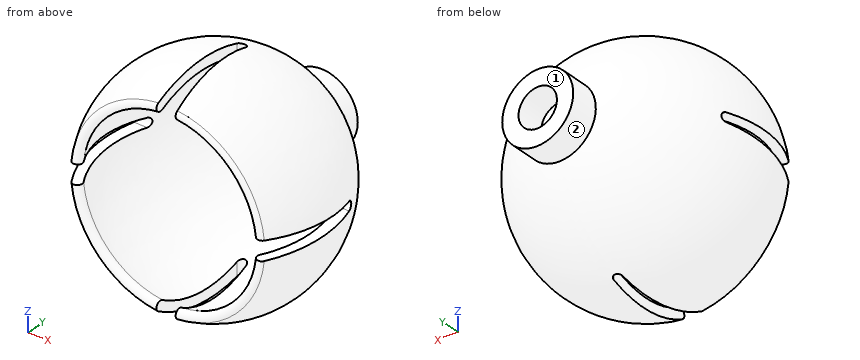
```python
from build123d import *

# Parameters (mm, degrees)
SKETCH1_R           = 3.7
SKETCH1_R_2         = 2
BOSS_EXTRUDE1_DEPTH = 3
CUT_EXTRUDE1_DEPTH  = 12.79718581
CIRPATTERN1_COUNT   = 4


with BuildPart() as part:
    # Sketch1 → Boss-Extrude1 (new body)
    with BuildSketch(Plane(origin=(0, 0, 0), x_dir=(1, 0, 0), z_dir=(0, 1, 0))):
        Circle(SKETCH1_R)
        Circle(SKETCH1_R_2, mode=Mode.SUBTRACT)
    extrude(amount=BOSS_EXTRUDE1_DEPTH)

    # Sketch2 → Revolve1 (revolve)
    with BuildSketch(Plane(origin=(0, 0, 0), x_dir=(0, 0, -1), z_dir=(1, 0, 0))):
        with BuildLine():
            Line((0, 0), (3.7, 0))
            ThreePointArc((3.7, 0), (11.06716667, -7.226007618), (10.1, -17.5))
            ThreePointArc((10.1, -17.5), (9.414366099, -17.672933956), (9.241432142, -16.987300055))
            ThreePointArc((9.241432142, -16.987300055), (9.596057225, -7.167858517), (1.5, -1.6))
            Line((1.5, -1.6), (1.5, -2.8))
            Line((1.5, -2.8), (0, -2.8))
            Line((0, -2.8), (0, 0))
        make_face()
    revolve(axis=Axis((0, 0, 0), (0, -1, 0)))

    # Sketch3 → Cut-Extrude1 (cut, symmetric)
    with BuildSketch(Plane(origin=(0, 0, 0), x_dir=(0, 0, -1), z_dir=(1, 0, 0))):
        with BuildLine():
            Line((-1, -17.743650027), (1, -17.743650027))
            Line((1, -17.743650027), (0.474618631, -7.718776319))
            ThreePointArc((0.474618631, -7.718776319), (0, -7.268380055), (-0.474618631, -7.718776319))
            Line((-0.474618631, -7.718776319), (-1, -17.743650027))
        make_face()
    cut_extrude1 = extrude(amount=CUT_EXTRUDE1_DEPTH, both=True, mode=Mode.SUBTRACT)

    # CirPattern1: Cut-Extrude1 ×4 about axis
    cirpattern1_axis = Axis((0, 0, 0), (0, 1, 0))
    for i in range(1, CIRPATTERN1_COUNT):
        add(cut_extrude1.rotate(cirpattern1_axis, i * 360 / CIRPATTERN1_COUNT), mode=Mode.SUBTRACT)


solid = part.part
```
Build history of the part. All positions in model axes, mm. Face numbers are marked on the shaded views. A direction names the side the tool comes from. Give positions to 0.01 mm unless a question says otherwise; leave off trailing zeros. Use a Markdown table: item, result.
(1) Wall check: line 1 along X through (y, z) = (2.3, 0); line 2 along Z through (x, y) = (-6.5, -7.75). Give the ranges that are in metal, low to high.
Taken from the geometry:
| item | result |
|---|---|
| line 1 | -3.7 to -2, 2 to 3.7 |
| line 2 | -9.18 to -7.42, 7.42 to 9.18 |
(2) Band-saw the part on A-A (y = -14.5). Give the number of separate pieces and of enclosed holes in the cut face, and give its area (3 significant figures).
Taken from the geometry:
| item | result |
|---|---|
| separate pieces | 4 |
| enclosed holes | 0 |
| area | 65.6 mm2 |
(3) Which spindle directions (+Z, -Z, +X, -X, +Y, -Y) get a long thin tool onto all of the face, cutting with end or side? Do the marked faces 1 and 2. Say none if no direction does.
Taken from the geometry:
| item | result |
|---|---|
| face 1 | +Z, -Z, +X, -X, +Y |
| face 2 | +Y |
(4) Drop flat-ended pins along their axis: pin 1 Ø10 at (y, z) = (-5, -7) entering from -X; pin 2 Ø3 at (x, z) = (0, 0) entering from -Y; pin 3 Ø1.5 at (x, y) = (-4, -2.5) entering from +Z. Give the stop position or say it passes through.
Taken from the geometry:
| item | result |
|---|---|
| pin 1 | x = -10.93 |
| pin 2 | y = -2.8 |
| pin 3 | z = 7.76 |
